from build123d import *

# Parameters (mm, degrees)
SKETCH1_R           = 36
SKETCH1_R_2         = 5
SKETCH1_R_3         = 21
SKETCH1_R_4         = 3
BOSS_EXTRUDE1_DEPTH = 10
SKETCH1_3_R         = 3
BOSS_EXTRUDE2_DEPTH = 40
LPATTERN3_COUNT     = 2
LPATTERN3_PITCH     = 30
SKETCH2_R           = 21
BOSS_EXTRUDE3_DEPTH = 10
SKETCH4_R           = 5
BOSS_EXTRUDE4_DEPTH = 20
FILLET1_R           = 10


with BuildPart() as part:
    # Sketch1 → Boss-Extrude1 (new body)
    with BuildSketch(Plane(origin=(0, 0, 0), x_dir=(1, 0, 0), z_dir=(0, 1, 0))):
        with Locations(Location((0, 0, 0), (0, 0, 270))):
            Circle(SKETCH1_R)
        with Locations(Location((0, 28.5, 0), (0, 0, 270))):
            Circle(SKETCH1_R_2, mode=Mode.SUBTRACT)
        with Locations(Location((24.681724008, -14.25, 0), (0, 0, 270))):
            Circle(SKETCH1_R_2, mode=Mode.SUBTRACT)
        with Locations(Location((-24.681724008, -14.25, 0), (0, 0, 270))):
            Circle(SKETCH1_R_2, mode=Mode.SUBTRACT)
        with Locations(Location((0, 0, 0), (0, 0, 270))):
            Circle(SKETCH1_R_3, mode=Mode.SUBTRACT)
        with Locations(Location((0, -28.5, 0), (0, 0, 270))):
            Circle(SKETCH1_R_4, mode=Mode.SUBTRACT)
        with Locations(Location((-24.681724008, 14.25, 0), (0, 0, 270))):
            Circle(SKETCH1_R_4, mode=Mode.SUBTRACT)
        with Locations(Location((24.681724008, 14.25, 0), (0, 0, 270))):
            Circle(SKETCH1_R_4, mode=Mode.SUBTRACT)
    boss_extrude1 = extrude(amount=BOSS_EXTRUDE1_DEPTH)

    # Sketch1_3 → Boss-Extrude2 (add)
    with BuildSketch(Plane(origin=(0, 0, 0), x_dir=(1, 0, 0), z_dir=(0, 1, 0))):
        with Locations(Location((0, -28.5, 0), (0, 0, 270))):
            Circle(SKETCH1_3_R)
        with Locations(Location((-24.681724008, 14.25, 0), (0, 0, 270))):
            Circle(SKETCH1_3_R)
        with Locations(Location((24.681724008, 14.25, 0), (0, 0, 270))):
            Circle(SKETCH1_3_R)
    extrude(amount=BOSS_EXTRUDE2_DEPTH)

    # LPattern3: Boss-Extrude1 ×2
    with Locations(*[(0, i * LPATTERN3_PITCH, 0) for i in range(1, LPATTERN3_COUNT)]):
        add(boss_extrude1)

    # Sketch2 → Boss-Extrude3 (add)
    with BuildSketch(Plane.XZ):
        with Locations(Location((0, 0, 0), (0, 0, 90))):
            Circle(SKETCH2_R)
    extrude(amount=-BOSS_EXTRUDE3_DEPTH)

    # Sketch4 → Boss-Extrude4 (add)
    with BuildSketch(Plane.XZ):
        with Locations(Location((0, 0, 0), (0, 0, 90))):
            Circle(SKETCH4_R)
    extrude(amount=BOSS_EXTRUDE4_DEPTH)

    # Fillet1
    fillet1_edges = [part.edges().sort_by_distance(p)[0] for p in [
        (0, 0, -5),
    ]]
    fillet(fillet1_edges, radius=FILLET1_R)


solid = part.part
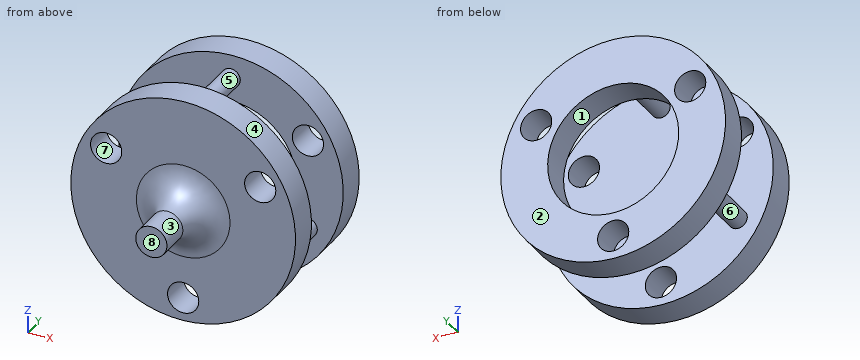
Can you work these out from the model? Positions are in its coordinate system, mm. Face numbers are marked on the shaded views. A direction names the side the tool comes from. Give positions to 0.01 mm unless a question says otherwise; leave off trailing zeros. Order: outer loops, then holes, each group sorted by start corner. A loop starts at its lowest first (then second) coordinate and runs counter-clockwise, first axis right, second up. Notation, with made-up numbers: M 37.5,77 L 76.5,77 A10 ccw 76.5,83 Z; hole C -16.75,42.25 d3. An arc over 180 degrees is marked long. Use one line per item in the form item = value. Start each with the question number.
Item 1: If we section it at C-C (z = -31): Write out the boundary of the cut face in (x, y).
Item 2: If I drill on line 1 along Y through (x, z) = (-15, -27); line 2 along X through (y, z) = (36, 0); line 3 along X through (y, z) = (6, 14), over which ranges is the centre line in solid material (lowest first)?
Item 3: If we section it at B-B (z = 0): Write out the boundary of the cut face in (x, y), then the cut area to 3 significant figures.
Item 4: Will these pins go through, and if not, where does the flat tip stop? pin 1 Ø1.5 at (y, z) = (29.5, -20) entering from -X; pin 2 Ø8 at (x, y) = (-22.5, 24) entering from -Z; pin 3 Ø12 at (y, z) = (5.5, -6.5) entering from +X; pin 4 Ø16 at (x, z) = (0, -28.5) entering from +Y.
Item 5: If we section it at D-D (x = 26.5): Write out the boundary of the cut face in (y, z), then the cut area to 3 significant figures.
Item 6: If we section it at A-A (x = 0): State how many separate pieces and enclosed holes the cut face has, then the cut area to 3 significant figures.
Item 7: For the marked faces 1, 2, 3, 4 and 5, which set-ups out of +Z, -Z, +X, -X, +Y, -Y let a thin tool reach every point of the face, with its end or its side?
Item 8: We'd pull the mould along Z, two halves only. Please class the marked faces 6, 7 and 8: +Z half, -Z half, draft (parallel to the pull), parting line (faces both ways), or undercut.
Outcome:
q1.outline = M -18.3,0 L -4.33,0 L -4.33,10 L -18.3,10 Z; M -18.3,30 L -4.33,30 L -4.33,40 L -18.3,40 Z; M 4.33,0 L 18.3,0 L 18.3,10 L 4.33,10 Z; M 4.33,30 L 18.3,30 L 18.3,40 L 4.33,40 Z
q2.line_1 = 0 to 10, 30 to 40
q2.line_2 = -36 to -21, 21 to 36
q2.line_3 = -33.17 to -29.68, -19.69 to 19.69, 29.68 to 33.17
q3.outline = M -36,0 L -15,0 A10 cw -5,-10 L -5,-20 L 5,-20 L 5,-10 A10 cw 15,0 L 36,0 L 36,10 L -36,10 Z; M -36,30 L -21,30 L -21,40 L -36,40 Z; M 21,30 L 36,30 L 36,40 L 21,40 Z
q3.area = 1,260 mm2
q4.pin_1 = -30.3
q4.pin_2 = -17.25
q4.pin_3 = 36
q4.pin_4 = 40
q5.outline = M 0,-24.37 L 10,-24.37 L 10,-16.64 L 30,-16.64 L 30,-24.37 L 40,-24.37 L 40,9.59 L 30,9.59 L 30,-11.86 L 10,-11.86 L 10,9.59 L 0,9.59 Z; M 0,18.91 L 10,18.91 L 10,24.37 L 0,24.37 Z; M 30,18.91 L 40,18.91 L 40,24.37 L 30,24.37 Z
q5.area = 884 mm2
q6.separate_pieces = 4
q6.enclosed_holes = 0
q6.area = 1,180 mm2
q7.face_1 = +Y
q7.face_2 = +Z, -Z, +X, -X, +Y
q7.face_3 = -Y
q7.face_4 = +Y, -Y
q7.face_5 = none
q8.face_6 = parting line
q8.face_7 = undercut
q8.face_8 = draft
